Input: part model. Units: mm. Frame: model coordinates. Face numbers are marked on the shaded views. A direction names the side the tool comes from. Give positions to 0.01 mm unless a question says otherwise; leave off trailing zeros. Write each loop counter-clockwise with the first axis right and the second up, starting at its lowest first coordinate (ties: lowest second). Pieces come first, ordered by that corner, then holes. Notation, with made-up numbers: (-2, 46) -> (48, 46) arc R28 cw to (48, 85) -> close; hole circle Ø8 at (75.25, 19.5). An arc over 180 degrees is marked (long way). Return JSON: item names as keys, results as strings. Group by question number.
Item 1: Pin query (flat end, axial travel): P1, Ø0.6, axis at x = -1.5, z = -7.5, coming from the +Y side; P2, Ø0.6, axis at y = 0, z = -12.5, coming from the -X side; P3, Ø1.5, axis at y = 2, z = -8, coming from the -X side. Return the tip coordinate at first contact, or that it passes through.
Item 2: Section C-C, the plane y = -1.8. Return loops of the section in (x, z).
Item 3: Line query: line 1 (X direction, y = 0.1, z = -2.5); line 2 (Z direction, x = -1.85, y = -0.95); line 3 (Y direction, x = 1.2, z = -18.5). Output: solid intervals per line, ascending. Write a range as [from, to].
Item 4: Set-up query: the marked faces 1 and 2. Return all of +Z, -Z, +X, -X, +Y, -Y with unobstructed straight access to the full face (end or side cutting, diameter ignored); none if empty.
Item 5: Section B-B, the plane x = -2. Return loops of the section in (y, z).
Item 6: Section A-A, the plane z = -18.5. Return loops of the section in (x, y).
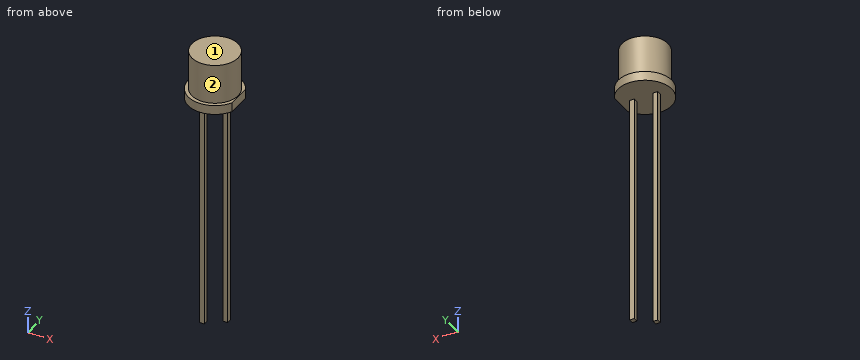
from build123d import *

# Parameters (mm, degrees)
PAD_DEPTH    = 1
SKETCH001_R  = 2.5
PAD001_DEPTH = 4.3
SKETCH002_W  = 0.5
SKETCH002_H  = 0.5
PAD002_DEPTH = 26
SKETCH003_W  = 0.5
SKETCH003_H  = 0.5
PAD003_DEPTH = 25


with BuildPart() as part:
    # Sketch → Pad (new body)
    with BuildSketch(Plane.XY):
        with BuildLine():
            ThreePointArc((2.58229, 1.319765), (-2.9, 0), (2.58229, -1.319765))
            Line((2.58229, -1.319765), (2.58229, 1.319765))
        make_face()
    extrude(amount=PAD_DEPTH)

    # Sketch001 (on Face4 of Pad) → Pad001 (join)
    with BuildSketch(Plane.XY.offset(1)):
        Circle(SKETCH001_R)
    extrude(amount=PAD001_DEPTH)

    # Sketch002 (on Face3 of Pad001) → Pad002 (join)
    with BuildSketch(Plane(origin=(0, 0, 0), x_dir=(1, 0, 0), z_dir=(0, 0, -1))):
        with Locations((-1.27, 0)):
            Rectangle(SKETCH002_W, SKETCH002_H)
    extrude(amount=PAD002_DEPTH)

    # Sketch003 (on Face3 of Pad002) → Pad003 (join)
    with BuildSketch(Plane(origin=(0, 0, 0), x_dir=(1, 0, 0), z_dir=(0, 0, -1))):
        with Locations((1.27, 0)):
            Rectangle(SKETCH003_W, SKETCH003_H)
    extrude(amount=PAD003_DEPTH)


solid = part.part
Answer below:
{
 "1": {"P1": "stops at y = 0.25", "P2": "stops at x = -1.52", "P3": "passes through"},
 "2": {"outline": "(-2.27, 0) -> (2.27, 0) -> (2.27, 1) -> (1.73, 1) -> (1.73, 5.3) -> (-1.73, 5.3) -> (-1.73, 1) -> (-2.27, 1) -> close"},
 "3": {"line 1": "x = [-1.52, -1.02], [1.02, 1.52]", "line 2": "z = [0, 5.3]", "line 3": "y = [-0.25, 0.25]"},
 "4": {"face 1": "+Z, +X, -X, +Y, -Y", "face 2": "+Z"},
 "5": {"outline": "(-2.1, 0) -> (2.1, 0) -> (2.1, 1) -> (1.5, 1) -> (1.5, 5.3) -> (-1.5, 5.3) -> (-1.5, 1) -> (-2.1, 1) -> close"},
 "6": {"outline": "(-1.52, -0.25) -> (-1.02, -0.25) -> (-1.02, 0.25) -> (-1.52, 0.25) -> close; (1.02, -0.25) -> (1.52, -0.25) -> (1.52, 0.25) -> (1.02, 0.25) -> close"}
}
